Read the model definition and answer for the solid it produces. Units are mm, in the model's axes. A direction names the side the tool comes from. Coordinates: 2 decimals unless noted, no trailing zeros. Loops run counter-clockwise (first coordinate to the right, second up) from the corner with the lowest first, then second, coordinate; pieces in that order, holes last. Notation, with made-up numbers: (-17.5, -21) -> (14.5, -21) arc R17 cw to (14.5, -10) -> close; hole circle Ø3 at (11.25, -2.75). An arc over 180 degrees is marked (long way). Answer as a JSON object with one key per item and string values. Group by question number.
1) Which of the six approach directions +Z, -Z, +X, -X, +Y, -Y give full straight-line access (tool end or side, diameter ignored) to faces 1 (the face through (-1.972, 11.855, 1.331)), 2 (the face through (2.51, 12.8, 4.31)), 3 (the face through (0.674, 12.17, -1.937))?
2) Section B-B, the plane x = 3 is taken. Give the vertices of the cut face in (y, z) (3 decimals).
3) Flat-ended cylindrical pins translate along their axes: P1, Ø3, axis at x = 1, y = 6.5, coming from the +Z side; P2, Ø1.4, axis at y = 12.2, z = -3.5, coming from the -X side; P3, Ø0.8, axis at x = 0, y = 12.2, coming from the -Z side. Find the tip coordinate at first contact, or state that the pin passes through.
4) Section A-A, the plane y = 5.6 is taken. Give the vertices of the cut face in (x, z).
5) Section C-C, the plane x = -1 is taken. Give the vertices of the cut face in (y, z), plus the area to 3 significant figures.
6) Section D-D, the plane y = 12.2 is taken. Give the vertices of the cut face in (x, z) (3 decimals), plus the area to 3 significant figures.
7) Consider probe 1 along Y at (x, z) = (0, 2.65); probe 2 along Z at (x, y) = (-1.7, 12.2); probe 3 along Y at (x, z) = (0, 3.8). Determine where each line is inside the solid, lowest interval first. Write a range as [from, to].
8) Determine the mould class of faces 4 (the face through (0, 4, 4.5)), 5 (the face through (0, 15, 0)), 6 (the face through (0, 12, 6.5)) for opening direction Y: released by +Y, released by -Y, zero draft, split by the parting line, or undercut.
from build123d import *

# Parameters (mm, degrees)
SKETCH1_W           = 7
SKETCH1_H           = 13
BOSS_EXTRUDE1_DEPTH = 15
SKETCH9_W           = 2
SKETCH9_H           = 7.2
CUT_EXTRUDE6_DEPTH  = 18.783419244
SKETCH20_R          = 1.35
CUT_EXTRUDE13_DEPTH = 19.927493231
SKETCH21_R          = 2.4
CUT_EXTRUDE14_DEPTH = 8
FILLET1_R           = 0.5
SKETCH17_R          = 0.675
SKETCH19_R          = 0.9
CUT_EXTRUDE12_DEPTH = 4
SKETCH22_W          = 5.5
SKETCH22_H          = 9.2
CUT_EXTRUDE15_DEPTH = 18.78341932


with BuildPart() as part:
    # Sketch1 → Boss-Extrude1 (new body)
    with BuildSketch(Plane(origin=(0, 0, 0), x_dir=(1, 0, 0), z_dir=(0, 1, 0))):
        Rectangle(SKETCH1_W, SKETCH1_H)
    extrude(amount=BOSS_EXTRUDE1_DEPTH)

    # Sketch9 → Cut-Extrude6 (cut, through all)
    with BuildSketch(Plane.ZY.offset(3.5)):
        with Locations((5.5, 5.6)):
            Rectangle(SKETCH9_W, SKETCH9_H)
    extrude(amount=-CUT_EXTRUDE6_DEPTH, mode=Mode.SUBTRACT)

    # Sketch20 → Cut-Extrude13 (cut, through all)
    with BuildSketch(Plane.XY.offset(4.5)):
        with Locations((0, 5.6)):
            Circle(SKETCH20_R)
    extrude(amount=-CUT_EXTRUDE13_DEPTH, mode=Mode.SUBTRACT)

    # Sketch21 → Cut-Extrude14 (cut)
    with BuildSketch(Plane(origin=(0, 0, -6.5), x_dir=(-1, 0, 0), z_dir=(0, 0, -1))):
        with Locations((0, 5.6)):
            Circle(SKETCH21_R)
    extrude(amount=-CUT_EXTRUDE14_DEPTH, mode=Mode.SUBTRACT)

    # Fillet1
    fillet1_edges = [part.edges().sort_by_distance(p)[0] for p in [
        (0, 2, 4.5),
        (0, 9.2, 4.5),
    ]]
    fillet(fillet1_edges, radius=FILLET1_R)

    # Cut-Sweep1: sweep along a path in Sketch16
    with BuildLine(Plane(origin=(0, 12.2, 0), x_dir=(-1, 0, 0), z_dir=(0, -1, 0))) as cut_sweep1_path:
        Line((0, 6.5), (0, -2.5))
        ThreePointArc((0, -2.5), (-0.439339828, -3.560660172), (-1.5, -4))
        Line((-1.5, -4), (-3.5, -4))
    # Sketch17 → Cut-Sweep1 (sweep, cut)
    with BuildSketch(Plane(origin=(0, 0, -6.5), x_dir=(-1, 0, 0), z_dir=(0, 0, -1))):
        with Locations((0, 12.2)):
            Circle(SKETCH17_R)
    sweep(path=cut_sweep1_path.line, mode=Mode.SUBTRACT)

    # Sketch19 → Cut-Extrude12 (cut)
    with BuildSketch(Plane.ZY.offset(3.5)):
        with Locations((0.5, 12.2)):
            Circle(SKETCH19_R)
        with Locations((-3.5, 12.2)):
            Circle(SKETCH19_R)
    extrude(amount=-CUT_EXTRUDE12_DEPTH, mode=Mode.SUBTRACT)

    # Sketch22 → Cut-Extrude15 (cut, through all)
    with BuildSketch(Plane(origin=(3.5, 0, 0), x_dir=(0, 0, -1), z_dir=(1, 0, 0))):
        with Locations((3.75, 4.6)):
            Rectangle(SKETCH22_W, SKETCH22_H)
    extrude(amount=-CUT_EXTRUDE15_DEPTH, mode=Mode.SUBTRACT)


solid = part.part
Determined:
{
 "1": {"face 1": "-X", "face 2": "+X", "face 3": "-Z"},
 "2": {"outline": "(0, -1) -> (9.2, -1) -> (9.2, -6.5) -> (15, -6.5) -> (15, 6.5) -> (9.2, 6.5) -> (9.2, 5) arc R0.5 cw to (8.7, 4.5) -> (2.5, 4.5) arc R0.5 cw to (2, 5) -> (2, 6.5) -> (0, 6.5) -> close; hole circle Ø1.35 at (12.2, 4)"},
 "3": {"P1": "z = 4.5", "P2": "x = 0.5", "P3": "z = 3.56"},
 "4": {"outline": "(-3.5, -1) -> (-2.4, -1) -> (-2.4, 1.5) -> (-1.35, 1.5) -> (-1.35, 4.5) -> (-3.5, 4.5) -> close; (1.35, 1.5) -> (2.4, 1.5) -> (2.4, -1) -> (3.5, -1) -> (3.5, 4.5) -> (1.35, 4.5) -> close"},
 "5": {"outline": "(0, -1) -> (3.42, -1) -> (3.42, 1.5) -> (4.69, 1.5) -> (4.69, 4.5) -> (2.5, 4.5) arc R0.5 cw to (2, 5) -> (2, 6.5) -> (0, 6.5) -> close; (6.51, 1.5) -> (7.78, 1.5) -> (7.78, -1) -> (9.2, -1) -> (9.2, -6.5) -> (15, -6.5) -> (15, 6.5) -> (9.2, 6.5) -> (9.2, 5) arc R0.5 cw to (8.7, 4.5) -> (6.51, 4.5) -> close; hole circle Ø1.8 at (12.2, -3.5); hole circle Ø1.8 at (12.2, 0.5)", "area": "109 mm²"},
 "6": {"outline": "(-3.5, -6.5) -> (-0.675, -6.5) -> (-0.675, -4.4) -> (-3.5, -4.4) -> close; (-3.5, -2.6) -> (-0.675, -2.6) -> (-0.675, -0.4) -> (-3.5, -0.4) -> close; (-3.5, 1.4) -> (-0.675, 1.4) -> (-0.675, 2.5) arc R2.175 cw to (1.5, 4.675) -> (3.5, 4.675) -> (3.5, 6.5) -> (-3.5, 6.5) -> close; (0.675, -6.5) -> (3.5, -6.5) -> (3.5, 3.325) -> (1.5, 3.325) arc R0.825 ccw to (0.675, 2.5) -> close", "area": "62.8 mm²"},
 "7": {"probe 1": "[0, 4.25], [6.95, 11.53], [12.87, 15]", "probe 2": "[-6.5, -4.4], [-2.6, -0.4], [1.4, 6.5]", "probe 3": "[0, 4.25], [6.95, 11.73], [12.67, 15]"},
 "8": {"face 4": "undercut", "face 5": "released by +Y", "face 6": "zero draft"}
}
